The model under review builds one solid part; all positions refer to its coordinate system, in mm. A direction names the side the tool comes from. Round coordinates to 2 decimals unless told otherwise and drop trailing zeros. Order: outer loops, then holes, each group sorted by start corner. A loop starts at its lowest first (then second) coordinate and runs counter-clockwise, first axis right, second up. Notation, with made-up numbers: M 69,19.5 L 123,19.5 A23 cw 123,52.5 Z; hole C 54,88.5 d1. An arc over 180 degrees is marked long. One line per item, written item: value. Start each with the question number.
from build123d import *

# Parameters (mm, degrees)
EXTRUDE_2_DEPTH     = 96
CHAMFER_1_SIZE      = 2
SKETCH_5_R          = 3
CUT_EXTRUDE_1_DEPTH = 12
CHAMFER_2_SIZE      = 2


with BuildPart() as part:
    # 草图4 → 拉伸2 (new body)
    with BuildSketch(Plane(origin=(0, -48, 0), x_dir=(-1, 0, 0), z_dir=(0, 1, 0))):
        with BuildLine():
            Line((7.833333333, 21), (-7.833333333, 21))
            Line((-7.833333333, 21), (-7.833333333, 23))
            Line((-7.833333333, 23), (-23, 23))
            Line((-23, 23), (-23, 12))
            Line((-23, 12), (-21, 10))
            Line((-21, 10), (-21, -16))
            Line((-21, -16), (-9.237604307, -16))
            Line((-9.237604307, -16), (-5, -8.660254038))
            ThreePointArc((-5, -8.660254038), (0, 10), (5, -8.660254038))
            Line((5, -8.660254038), (9.237604307, -16))
            Line((9.237604307, -16), (22, -16))
            Line((22, -16), (22, 10))
            Line((22, 10), (24, 12))
            Line((24, 12), (24, 23))
            Line((24, 23), (7.833333333, 23))
            Line((7.833333333, 23), (7.833333333, 21))
        make_face()
    extrude(amount=EXTRUDE_2_DEPTH)

    # 倒角1
    chamfer_1_edges = [part.edges().sort_by_distance(p)[0] for p in [
        (-7.833333333, 0, 23),
        (7.833333333, 0, 23),
    ]]
    chamfer(chamfer_1_edges, length=CHAMFER_1_SIZE - 0.0001)  # a hair under: the kernel refuses the full size

    # 草图5 → 切除-拉伸1 (cut)
    with BuildSketch(Plane.XY.offset(23)):
        with Locations((-18, 35)):
            Circle(SKETCH_5_R)
        with Locations((17, 35)):
            Circle(SKETCH_5_R)
        with Locations((17, -35)):
            Circle(SKETCH_5_R)
        with Locations((-18, -35)):
            Circle(SKETCH_5_R)
    extrude(amount=-CUT_EXTRUDE_1_DEPTH, mode=Mode.SUBTRACT)

    # 倒角2
    chamfer_2_edges = [part.edges().sort_by_distance(p)[0] for p in [
        (-22, 0, -16),
        (21, 0, -16),
    ]]
    chamfer(chamfer_2_edges, length=CHAMFER_2_SIZE)

    # 草图6 → 切除-旋转1 (revolve, cut)
    with BuildSketch(Plane(origin=(0, 0, 0), x_dir=(0, 0, -1), z_dir=(1, 0, 0))):
        with BuildLine():
            Line((-16.2, -48), (-16, -47.8))
            ThreePointArc((-16, -47.8), (-15.940621125, -47.941496067), (-15.798761062, -48))
            Line((-15.798761062, -48), (-16.2, -48))
        make_face()
        with BuildLine():
            Line((-15.45, -48), (0, -48))
            Line((0, -48), (0, -47.8))
            Line((0, -47.8), (-15.25, -47.8))
            ThreePointArc((-15.25, -47.8), (-15.308578644, -47.941421356), (-15.45, -48))
        make_face()
    cut_revolve_1 = revolve(axis=Axis((0, -10.264906919, 0), (0, -1, 0)), mode=Mode.SUBTRACT)

    # 镜向1: 切除-旋转1 across plane
    add(cut_revolve_1.mirror(Plane.ZX), mode=Mode.SUBTRACT)


solid = part.part
Item 1: Consider section A-A, the plane z = 0. Give the boundary of the cut face in (x, y), then the cut area to 3 significant figures.
Item 2: Wall thickness on L1, parallel to Y at x = -18, z = 14.5; L2, parallel to Z at x = 0, y = -25; L3, parallel to Z at x = 5.5, y = -5: over which ranges is each line inside the solid? List them lowest first.
Item 3: Clearance check with flat-ended pins moving along their axes: P1, Ø4, axis at y = -22, z = -7, coming from the -X side; P2, Ø1.8, axis at x = -18.5, y = -34.5, coming from the +Z side; P3, Ø4.5, axis at x = -2, y = -14, coming from the +Z side. State where each tip first meets the part, or that it passes through.
Item 4: Machinability: for faces 4 (the flat face through (21, -1, -2)), 5 (the flat face through (0, -1, 21)), 6 (the cylindrical face through (-20.21, 37.03, 17.08)), 7 (the flat face through (0, 47.8, 11)), 8 (the flat face through (-7.1, -0.7, -12.3)), which of the approach directions +Z, -Z, +X, -X, +Y, -Y give a long, thin tool a straight path to every point of the face, cutting with its end or side? Answer none if there is none.
Item 5: The part is to be moulded in two halves that separate along Y. For faces 1 (the flat face through (22, -1, 11)), 2 (the flat face through (-18, 35, 11)), 3 (the flat face through (0, 48, 17)), say which applies: pulls with the +Y half, pulls with the -Y half, needs draft (parallel to the pull), parting line crosses it, or undercut.
Item 6: Consider section B-B, the plane x = 0. Give the boundary of the cut face in (y, z), then the cut area to 3 significant figures.
Computed:
1. outline: M -22,-48 L -16.2,-48 L -16,-47.8 A0.2 ccw -15.8,-48 L -15.45,-48 A0.2 ccw -15.25,-47.8 L -10,-47.8 L -10,47.8 L -15.25,47.8 A0.2 ccw -15.45,48 L -15.8,48 A0.2 ccw -16,47.8 L -16.2,48 L -22,48 Z; M 10,-47.8 L 15.25,-47.8 A0.2 ccw 15.45,-48 L 15.8,-48 A0.2 ccw 16,-47.8 L 16.2,-48 L 21,-48 L 21,48 L 16.2,48 L 16,47.8 A0.2 ccw 15.8,48 L 15.45,48 A0.2 ccw 15.25,47.8 L 10,47.8 Z
1. area: 2,200 mm^2
2. L1: y = -48 to -38, -32 to 32, 38 to 48
2. L2: z = 10 to 21
2. L3: z = -9.53 to -8.35, 8.35 to 21
3. P1: stops at x = -22
3. P2: stops at z = 11
3. P3: stops at z = 21
4. face 4: -Z, +X, +Y, -Y
4. face 5: +Z, +Y, -Y
4. face 6: +Z
4. face 7: +Y
4. face 8: -Z, +Y, -Y
5. face 1: needs draft
5. face 2: undercut
5. face 3: pulls with the +Y half
6. outline: M -48,15.45 A0.2 ccw -47.8,15.25 L -47.8,10 L 47.8,10 L 47.8,15.25 A0.2 ccw 48,15.45 L 48,15.8 A0.2 ccw 47.8,16 L 48,16.2 L 48,21 L -48,21 L -48,16.2 L -47.8,16 A0.2 ccw -48,15.8 Z
6. area: 1,050 mm^2
